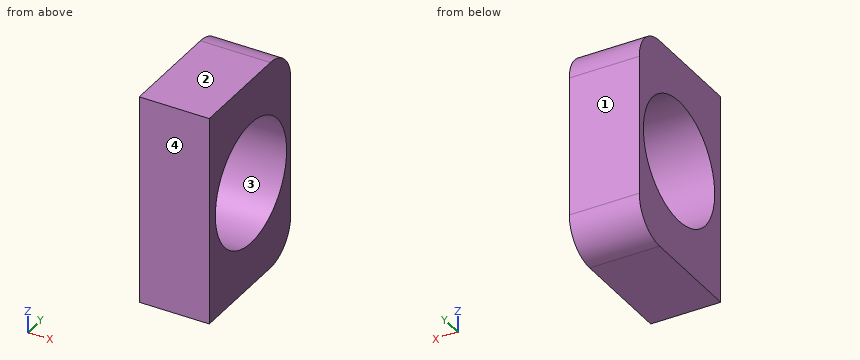
```python
from build123d import *

# Parameters (mm, degrees)
SKETCH1_W           = 12.7
SKETCH1_H           = 38.1
BOSS_EXTRUDE1_DEPTH = 25.4
FILLET1_R           = 6.35
SKETCH2_R           = 11.1125
CUT_EXTRUDE1_DEPTH  = 13.7


with BuildPart() as part:
    # Sketch1 → Boss-Extrude1 (new body)
    with BuildSketch(Plane(origin=(0, 0, 0), x_dir=(1, 0, 0), z_dir=(0, 1, 0))):
        Rectangle(SKETCH1_W, SKETCH1_H)
    extrude(amount=BOSS_EXTRUDE1_DEPTH)

    # Fillet1
    fillet1_edges = [part.edges().sort_by_distance(p)[0] for p in [
        (0, 25.4, 19.05),
        (0, 25.4, -19.05),
    ]]
    fillet(fillet1_edges, radius=FILLET1_R)

    # Sketch2 → Cut-Extrude1 (cut, through all)
    with BuildSketch(Plane.ZY.offset(6.35)):
        with Locations((0, 13)):
            Circle(SKETCH2_R)
    extrude(amount=-CUT_EXTRUDE1_DEPTH, mode=Mode.SUBTRACT)


solid = part.part
```
Could you check a few things on this model? Use its own coordinates, in mm. Face numbers are marked on the shaded views. Coordinates: 2 decimals unless noted, no trailing zeros. Loops run counter-clockwise (first coordinate to the right, second up) from the corner with the lowest first, then second, coordinate; pieces in that order, holes last. Notation, with made-up numbers: M 40,80 L 94,80 A13 ccw 94,97 Z; hole C 2,-9 d8. An arc over 180 degrees is marked long. Put each result on its own line as item: value. Start each with the question number.
(1) Suppose I cut it at D-D on z = 16.5. Please give me the cut outline in (x, y).
(2) Will this pin go through, and if not, where does the flat tip stop? P1, Ø2, axis at x = -1, y = 22, coming from the -Z side.
(3) Suppose I cut it at B-B on y = 10. Please give me the cut outline in (x, z), then the cut area to 3 significant figures.
(4) Thinking about a two-plate mould opening in Y: for the marked faces 1, 2, 3 and 4, which applies, pulls with the +Y half, pulls with the -Y half, needs draft (parallel to the pull), parting line crosses it, or undercut?
(5) I need wall thicknesses on line 1 (Y direction, x = 3.25, z = 0); line 2 (Z direction, x = 1, y = 20.75); line 3 (Z direction, x = 0.5, y = 12.25). Which ranges of each line are inside material? Lowest first, please. Write a range as from..to.
(6) Suppose I cut it at A-A on z = 0. Please give me the cut outline in (x, y).
Solutions:
1. outline: M -6.35,0 L 6.35,0 L 6.35,24.14 L -6.35,24.14 Z
2. P1: stops at z = -18.74
3. outline: M -6.35,-19.05 L 6.35,-19.05 L 6.35,-10.7 L -6.35,-10.7 Z; M -6.35,10.7 L 6.35,10.7 L 6.35,19.05 L -6.35,19.05 Z
3. area: 212 mm2
4. face 1: pulls with the +Y half
4. face 2: needs draft
4. face 3: undercut
4. face 4: pulls with the -Y half
5. line 1: y = 0..1.89, 24.11..25.4
5. line 2: z = -18.82..-7.96, 7.96..18.82
5. line 3: z = -19.05..-11.09, 11.09..19.05
6. outline: M -6.35,0 L 6.35,0 L 6.35,1.89 L -6.35,1.89 Z; M -6.35,24.11 L 6.35,24.11 L 6.35,25.4 L -6.35,25.4 Z
